Input: part model. Units: mm. Frame: model coordinates. Round coordinates to 2 decimals unless told otherwise and drop trailing zeros. Write each loop counter-clockwise with the first axis right and the second up, starting at its lowest first coordinate (ties: lowest second). Pieces come first, ordered by that corner, then holes. Notation, with made-up numbers: M -14.5,-12 L 17.5,-12 A16 cw 17.5,-7 Z; hole C 53.25,24 d3. An arc over 180 degrees is marked long. Answer as CSV lines item,"result". Start each with the question number.
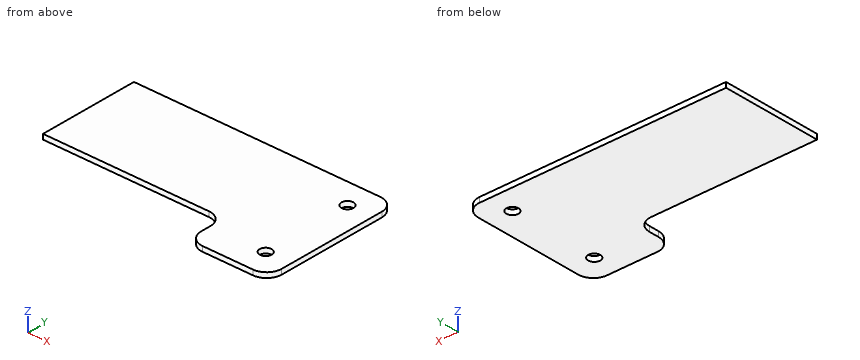
```python
from build123d import *

# Parameters (mm, degrees)
SKETCH1_R           = 6
BOSS_EXTRUDE1_DEPTH = 2.5


with BuildPart() as part:
    # Sketch1 → Boss-Extrude1 (new, symmetric)
    with BuildSketch(Plane.XY):
        with BuildLine():
            Line((-122.5, 70), (122.5, 70))
            ThreePointArc((122.5, 70), (133.106601718, 65.606601718), (137.5, 55))
            Line((137.5, 55), (137.5, -55))
            ThreePointArc((137.5, -55), (133.106601718, -65.606601718), (122.5, -70))
            Line((122.5, -70), (72.5, -70))
            ThreePointArc((72.5, -70), (61.893398282, -65.606601718), (57.5, -55))
            Line((57.5, -55), (57.5, -45))
            ThreePointArc((57.5, -45), (53.106601718, -34.393398282), (42.5, -30))
            Line((42.5, -30), (-122.5, -30))
            Line((-122.5, -30), (-122.5, 70))
        make_face()
        with Locations((112.5, 45)):
            Circle(SKETCH1_R, mode=Mode.SUBTRACT)
        with Locations(Location((112.5, -45, 0), (0, 0, 180))):
            Circle(SKETCH1_R, mode=Mode.SUBTRACT)
    extrude(amount=BOSS_EXTRUDE1_DEPTH, both=True)


solid = part.part
```
Item 1: Cut plane B-B, the plane y = 45. Return loops of the section in (x, z), plus the area to 3 significant figures.
Item 2: Cut plane C-C, the plane z = 0.5. Return loops of the section in (x, y).
Item 3: Line query: line 1 (Y direction, x = 112.5, z = -0.5); line 2 (X direction, y = -45, z = 1.1); line 3 (X direction, y = -55.5, z = 0.15). Output: solid intervals per line, ascending. Write a range as [from, to].
Item 4: Cut plane D-D, the plane x = 54.5. Return loops of the section in (y, z).
Item 5: Cut plane A-A, the plane x = 112.5. Return loops of the section in (y, z), plus the area to 3 significant figures.
Results list:
1,outline,"M -122.5,-2.5 L 106.5,-2.5 L 106.5,2.5 L -122.5,2.5 Z; M 118.5,-2.5 L 137.5,-2.5 L 137.5,2.5 L 118.5,2.5 Z"
1,area,"1,240 mm²"
2,outline,"M -122.5,-30 L 42.5,-30 A15 cw 57.5,-45 L 57.5,-55 A15 ccw 72.5,-70 L 122.5,-70 A15 ccw 137.5,-55 L 137.5,55 A15 ccw 122.5,70 L -122.5,70 Z; hole C 112.5,-45 d12; hole C 112.5,45 d12"
3,line 1,"[-70, -51], [-39, 39], [51, 70]"
3,line 2,"[57.5, 106.5], [118.5, 137.5]"
3,line 3,"[57.51, 137.49]"
4,outline,"M -36,-2.5 L 70,-2.5 L 70,2.5 L -36,2.5 Z"
5,outline,"M -70,-2.5 L -51,-2.5 L -51,2.5 L -70,2.5 Z; M -39,-2.5 L 39,-2.5 L 39,2.5 L -39,2.5 Z; M 51,-2.5 L 70,-2.5 L 70,2.5 L 51,2.5 Z"
5,area,"580 mm²"
